from build123d import *

# Parameters (mm, degrees)
BASPROSKE_W             = 5
BASPROSKE_H             = 13.5
TOOTHCUT_DEPTH          = 20.735754356
TEETHCUTS_COUNT         = 16
TEETHCUTS_ANGLE         = 337.5
BORSKE_R                = 2.5
BORE_DEPTH              = 50.0000508
ENL_V_MAT_EXTRU_1_DEPTH = 2
ESQUISSE2_R             = 0.5
ENL_V_MAT_EXTRU_2_DEPTH = 20.053559185


with BuildPart() as part:
    # BasProSke → Base-Revolve (revolve)
    with BuildSketch(Plane(origin=(0, 0, 0), x_dir=(1, 0, 0), z_dir=(0, 1, 0)), mode=Mode.PRIVATE) as base_revolve_sk:
        with Locations((2.5, 6.75)):
            Rectangle(BASPROSKE_W, BASPROSKE_H)
    revolve(base_revolve_sk.sketch.rotate(Axis((-10, 0, 0), (1, 0, 0)), 180), axis=Axis((-10, 0, 0), (1, 0, 0)))

    # TooCutSke → ToothCut (cut, through all)
    with BuildSketch(Plane(origin=(0, 0, 0), x_dir=(0, 0, -1), z_dir=(1, 0, 0))):
        with BuildLine():
            ThreePointArc((0.779807897, 10.093922708), (0, 10.124), (-0.779807897, 10.093922708))
            ThreePointArc((-0.779807897, 10.093922708), (-1.232785697, 11.858156262), (-2.310463203, 13.326597651))
            ThreePointArc((-2.310463203, 13.326597651), (0, 13.5254), (2.310463203, 13.326597651))
            ThreePointArc((2.310463203, 13.326597651), (1.232785697, 11.858156262), (0.779807897, 10.093922708))
        make_face()
    toothcut = extrude(amount=TOOTHCUT_DEPTH, mode=Mode.SUBTRACT)

    # TeethCuts: ToothCut ×16 about axis
    teethcuts_axis = Axis((-10, 0, 0), (1, 0, 0))
    for i in range(1, TEETHCUTS_COUNT):
        add(toothcut.rotate(teethcuts_axis, i * TEETHCUTS_ANGLE / (TEETHCUTS_COUNT - 1)), mode=Mode.SUBTRACT)

    # BorSke → Bore (cut, symmetric)
    with BuildSketch(Plane(origin=(0, 0, 0), x_dir=(0, 0, -1), z_dir=(1, 0, 0))):
        with Locations(Location((0, 0, 0), (0, 0, 180))):
            Circle(BORSKE_R)
    extrude(amount=BORE_DEPTH, both=True, mode=Mode.SUBTRACT)

    # Esquisse1 → Enlèv. mat.-Extru.1 (cut)
    with BuildSketch(Plane(origin=(5, 0, 0), x_dir=(0, 0, -1), z_dir=(1, 0, 0))):
        with BuildLine():
            Line((-6.353817175, -1.786479026), (-3.411680983, -1.792741804))
            Line((-3.411680983, -1.792741804), (-3.062404796, -5.643188497))
            ThreePointArc((-3.062404796, -5.643188497), (-0.017415965, -8.181695296), (3.038352407, -5.656174874))
            Line((3.038352407, -5.656174874), (3.404017861, -1.80725004))
            Line((3.404017861, -1.80725004), (6.346154052, -1.813512818))
            ThreePointArc((6.346154052, -1.813512818), (8.149981536, -0.017348458), (6.353817175, 1.786479026))
            Line((6.353817175, 1.786479026), (3.411680983, 1.792741804))
            Line((3.411680983, 1.792741804), (3.062404796, 5.643188497))
            ThreePointArc((3.062404796, 5.643188497), (0.017415965, 8.181695296), (-3.038352407, 5.656174874))
            Line((-3.038352407, 5.656174874), (-3.404017861, 1.80725004))
            Line((-3.404017861, 1.80725004), (-6.346154052, 1.813512818))
            ThreePointArc((-6.346154052, 1.813512818), (-8.149981536, 0.017348458), (-6.353817175, -1.786479026))
        make_face()
    extrude(amount=-ENL_V_MAT_EXTRU_1_DEPTH, mode=Mode.SUBTRACT)

    # Esquisse2 → Enlèv. mat.-Extru.2 (cut, through all)
    with BuildSketch(Plane(origin=(3, 0, 0), x_dir=(0, 0, -1), z_dir=(1, 0, 0))):
        with Locations((-0.010809829, -5.078255711)):
            Circle(ESQUISSE2_R)
        with Locations((0.010809829, 5.078255711)):
            Circle(ESQUISSE2_R)
    extrude(amount=-ENL_V_MAT_EXTRU_2_DEPTH, mode=Mode.SUBTRACT)


solid = part.part
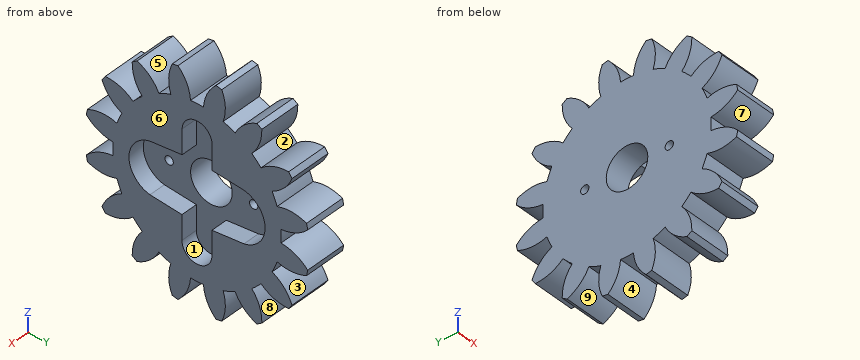
Could you check a few things on this model? Use its own coordinates, in mm. Face numbers are marked on the shaded views. A direction names the side the tool comes from. Give positions to 0.01 mm unless a question says otherwise; leave off trailing zeros. Order: outer loops, then holes, each group sorted by start corner. A loop starts at its lowest first (then second) coordinate and runs counter-clockwise, first axis right, second up. Notation, with made-up numbers: (12.5, 3) - (49.5, 3) arc R13 cw to (49.5, 15) - close; hole circle Ø11 at (-33, 50.25). An arc over 180 degrees is marked (long way). One line per item, written item: value. Start each with the question number.
1. Imagine slicing it at A-A on z = 0. List the corners of the cut face in (x, y) for me, plus the area to 3 significant figures.
2. Imagine slicing it at B-B on y = 0. List the corners of the cut face in (x, z) for me.
3. For P1, Ø3, axis at y = 3, z = 7, coming from the -X side; P2, Ø1, axis at x = 1, z = -5.5, coming from the -Y side, each with a flat end and sliding along its axis, tell me the tip position at first contact or that it passes through.
4. Imagine slicing it at D-D on x = 2.5. Give the number of separate pieces and of enclosed holes in the cut face, plus the area to 3 significant figures.
5. Imagine slicing it at C-C on y = 3.75. List the corners of the cut face in (x, z) for me.
6. For the marked faces 1, 2, 3, 4 and 5, which set-ups out of +Z, -Z, +X, -X, +Y, -Y let a thin tool reach every point of the face, with its end or its side?
7. If I drill on probe 1 along Z at (x, y) = (4.5, 10.75); probe 2 along Z at (x, y) = (3.5, -6.75); probe 3 along Y at (x, z) = (0.8, 11.25), over which ranges is the centre line in solid material (lowest first)?
8. Thinking about a two-plate mould opening in Z: for the marked faces 6, 7, 8 and 9, which applies, +Z half, -Z half, draft (parallel to the pull), parting line (faces both ways), or undercut?
Values:
1. outline: (0, -10.12) - (5, -10.12) - (5, -8.18) - (3, -8.18) - (3, -5.58) - (0, -5.58) - close; (0, -4.58) - (3, -4.58) - (3, -2.5) - (0, -2.5) - close; (0, 2.5) - (3, 2.5) - (3, 4.58) - (0, 4.58) - close; (0, 5.58) - (3, 5.58) - (3, 8.18) - (5, 8.18) - (5, 10.12) - (0, 10.12) - close
1. area: 47.5 mm²
2. outline: (0, -10.12) - (5, -10.12) - (5, -8.15) - (3, -8.15) - (3, -2.5) - (0, -2.5) - close; (0, 2.5) - (3, 2.5) - (3, 8.15) - (5, 8.15) - (5, 10.12) - (0, 10.12) - close
3. P1: x = 0
3. P2: y = -10.75
4. separate pieces: 1
4. enclosed holes: 3
4. area: 411 mm²
5. outline: (0, -9.4) - (5, -9.4) - (5, -3.23) - (3, -3.23) - (3, 3.22) - (5, 3.22) - (5, 9.4) - (0, 9.4) - close
6. face 1: +X
6. face 2: +X, -X
6. face 3: +X, -X, +Y
6. face 4: -Z, +X, -X
6. face 5: +Z, +X, -X
7. probe 1: -7.79 to -6, -3.38 to -0.87, 0.87 to 3.38, 6 to 7.79
7. probe 2: -11.22 to -7.88, -7.55 to -2.6, 2.63 to 7.55, 7.88 to 11.22
7. probe 3: -7.46 to -6.82, -3.4 to -0.99, 0.99 to 3.4, 6.82 to 7.46
8. face 6: draft
8. face 7: undercut
8. face 8: undercut
8. face 9: -Z half
